```python
from build123d import *

# Parameters (mm, degrees)
F0_R     = 1.2
F0_R_2   = 2.05
F1_DEPTH = 5.6


with BuildPart() as f1:
    # F0 (on Top) → F1 (new body)
    with BuildSketch(Plane.XY):
        with BuildLine():
            Line((31.5, 25.5), (39.5, 25.5))
            Line((39.5, 25.5), (39.5, 44.5))
            Line((39.5, 44.5), (22.808842361, 61.3844171166))
            Line((22.808842361, 61.3844171166), (0, 61.3844171166))
            Line((0, 61.3844171166), (-22.808842361, 61.3844171166))
            Line((-22.808842361, 61.3844171166), (-39.5, 44.5))
            Line((-39.5, 44.5), (-39.5, 25.5))
            Line((-39.5, 25.5), (-31.5, 25.5))
            Line((-31.5, 25.5), (-31.5, 18.901754251))
            ThreePointArc((-31.5, 18.901754251), (0, 41), (31.5, 18.901754251))
            Line((31.5, 18.901754251), (31.5, 25.5))
        make_face()
        with Locations((-35, 43)):
            Circle(F0_R, mode=Mode.SUBTRACT)
        with Locations((0, 54.8844171166)):
            Circle(F0_R_2, mode=Mode.SUBTRACT)
        with Locations((35, 43)):
            Circle(F0_R, mode=Mode.SUBTRACT)
        with BuildLine():
            ThreePointArc((-31.5, -3.901754251), (0, -26), (31.5, -3.901754251))
            Line((31.5, -3.901754251), (31.5, 18.901754251))
            ThreePointArc((31.5, 18.901754251), (0, 41), (-31.5, 18.901754251))
            Line((-31.5, 18.901754251), (-31.5, -3.901754251))
        make_face()
        with BuildLine():
            Line((22.808842361, -61.3844171166), (39.5, -44.5))
            Line((39.5, -44.5), (39.5, -9.5))
            Line((39.5, -9.5), (31.5, -9.5))
            Line((31.5, -9.5), (31.5, -3.901754251))
            ThreePointArc((31.5, -3.901754251), (0, -26), (-31.5, -3.901754251))
            Line((-31.5, -3.901754251), (-31.5, -9.5))
            Line((-31.5, -9.5), (-39.5, -9.5))
            Line((-39.5, -9.5), (-39.5, -44.5))
            Line((-39.5, -44.5), (-22.808842361, -61.3844171166))
            Line((-22.808842361, -61.3844171166), (0, -61.3844171166))
            Line((0, -61.3844171166), (22.808842361, -61.3844171166))
        make_face()
        with Locations((-35, -43)):
            Circle(F0_R, mode=Mode.SUBTRACT)
        with Locations((0, -54.8844171166)):
            Circle(F0_R_2, mode=Mode.SUBTRACT)
        with Locations((35, -43)):
            Circle(F0_R, mode=Mode.SUBTRACT)
    extrude(amount=F1_DEPTH)


solid = f1.part
```
Could you check a few things on this model? Use its own coordinates, in mm. A direction names the side the tool comes from. Round coordinates to 2 decimals unless told otherwise and drop trailing zeros. Loops run counter-clockwise (first coordinate to the right, second up) from the corner with the lowest first, then second, coordinate; pieces in that order, holes last. Notation, with made-up numbers: (-24.75, 80) - (25.25, 80) arc R34 ccw to (25.25, 112) - close; hole circle Ø1 at (-32.5, 75.25). An arc over 180 degrees is marked (long way). Answer in a Markdown table with one row per item. Add a question column.
(1) If we mould it in two halves opening along Y, with no side actions, what happens to faces 4 (the face through (0, -61.384, 3)), 5 (the face through (-1, 1, 5.6)), 6 (the face through (-35, -9.5, 3))? For each: pulls with the +Y half, pulls with the -Y half, needs draft (parallel to the pull), parting line crosses it, or undercut.
(2) For faces 1 (the face through (-36, 25.5, 3)), 2 (the face through (-0.444, -56.886, 2.761)), 3 (the face through (31.5, 8, 3)), which set-ups out of +Z, -Z, +X, -X, +Y, -Y let a thin tool reach every point of the face, with its end or its side?
(3) If we section it at B-B (y = -43): Please give me the cut outline in (x, z).
(4) If we section it at A-A (x = 0): Please give me the cut outline in (y, z).
(5) If we section it at C-C (z = 3.85): Please give me the cut outline in (x, y), plus the area to 3 significant figures.
(6) I need wall thicknesses on line 1 along Y through (x, z) = (0, 3.25); line 2 along Y through (x, z) = (-35, 2); line 3 along X through (y, z) = (12, 3.1). Which ranges of each line are inside material? Lowest first, please.
(7) If we section it at D-D (x = 35): Please give me the cut outline in (y, z).
(8) I'm going to push flat-ended pins straight in: pin 1 (1.5 mm diameter, centred on x = 7.5, y = -20.5, fed in from -Z); pin 2 (3 mm diameter, centred on x = 37, z = 4, fed in from +Y); pin 3 (3 mm diameter, centred on y = 2.5, z = 2, fed in from -X); pin 4 (1.7 mm diameter, centred on x = -35.5, z = 3, fed in from +Y). Where does each tip first touch, or does it pass through?
Model answer:
| question | item | result |
|---|---|---|
| 1 | face 4 | pulls with the -Y half |
| 1 | face 5 | needs draft |
| 1 | face 6 | undercut |
| 2 | face 1 | +Z, -Z, -X |
| 2 | face 2 | +Z, -Z |
| 2 | face 3 | +Z, -Z, +X |
| 3 | outline | (-39.5, 0) - (-36.2, 0) - (-36.2, 5.6) - (-39.5, 5.6) - close; (-33.8, 0) - (33.8, 0) - (33.8, 5.6) - (-33.8, 5.6) - close; (36.2, 0) - (39.5, 0) - (39.5, 5.6) - (36.2, 5.6) - close |
| 4 | outline | (-61.38, 0) - (-56.93, 0) - (-56.93, 5.6) - (-61.38, 5.6) - close; (-52.83, 0) - (52.83, 0) - (52.83, 5.6) - (-52.83, 5.6) - close; (56.93, 0) - (61.38, 0) - (61.38, 5.6) - (56.93, 5.6) - close |
| 5 | outline | (-39.5, -44.5) - (-22.81, -61.38) - (22.81, -61.38) - (39.5, -44.5) - (39.5, -9.5) - (31.5, -9.5) - (31.5, 25.5) - (39.5, 25.5) - (39.5, 44.5) - (22.81, 61.38) - (-22.81, 61.38) - (-39.5, 44.5) - (-39.5, 25.5) - (-31.5, 25.5) - (-31.5, -9.5) - (-39.5, -9.5) - close; hole circle Ø2.4 at (-35, -43); hole circle Ø2.4 at (-35, 43); hole circle Ø4.1 at (0, -54.88); hole circle Ø4.1 at (0, 54.88); hole circle Ø2.4 at (35, -43); hole circle Ø2.4 at (35, 43) |
| 5 | area | 8,530 mm² |
| 6 | line 1 | y = -61.38 to -56.93, -52.83 to 52.83, 56.93 to 61.38 |
| 6 | line 2 | y = -49.05 to -44.2, -41.8 to -9.5, 25.5 to 41.8, 44.2 to 49.05 |
| 6 | line 3 | x = -31.5 to 31.5 |
| 7 | outline | (-49.05, 0) - (-44.2, 0) - (-44.2, 5.6) - (-49.05, 5.6) - close; (-41.8, 0) - (-9.5, 0) - (-9.5, 5.6) - (-41.8, 5.6) - close; (25.5, 0) - (41.8, 0) - (41.8, 5.6) - (25.5, 5.6) - close; (44.2, 0) - (49.05, 0) - (49.05, 5.6) - (44.2, 5.6) - close |
| 8 | pin 1 | stops at z = 0 |
| 8 | pin 2 | stops at y = 48.55 |
| 8 | pin 3 | stops at x = -31.5 |
| 8 | pin 4 | stops at y = 49.41 |
